The model under review builds one solid part; all positions refer to its coordinate system, in mm. A direction names the side the tool comes from. Give positions to 0.01 mm unless a question says otherwise; leave off trailing zeros. Loops run counter-clockwise (first coordinate to the right, second up) from the corner with the lowest first, then second, coordinate; pieces in that order, holes last. Notation, with made-up numbers: M -8,68 L 18,68 A11 cw 18,77 Z; hole C 82,-16 d4. An arc over 180 degrees is marked long. Write item = value, one per line. Start each with the question number.
1. We need section C-C on x = 0. Give the boundary of the cut face in (y, z), then the cut area to 3 significant figures.
2. Wall thickness on line 1 along X through (y, z) = (5.5, -5); line 2 along Z through (x, y) = (-8.5, 7); line 3 along Z through (x, y) = (3.25, 4): over which ranges is each line inside the solid? List them lowest first. Write a range as from..to.
3. For pin 1 (5 mm diameter, centred on x = -7.5, z = -8.5, fed in from +Y); pin 2 (6 mm diameter, centred on x = 6.5, y = 11, fed in from +Z); pin 3 (3.5 mm diameter, centred on x = -13, z = 16, fed in from +Y); pin 4 (5 mm diameter, centred on y = 22, z = -0.5, fed in from -X), all flat-tipped, find the tip position at first contact; note any pin that passes through.
4. We need section A-A on y = 21. Give the boundary of the cut face in (x, z).
5. For faces 1 (the face through (4.4, 2, 1)), 2 (the face through (-13, 6.8, 15)), 3 (the face through (-11, 13, -5)), list the 3-axis set-ups (+Z, -Z, +X, -X, +Y, -Y) from which the entire face can be reached by the end or side of a thin tool; tool diameter is ignored.
6. We need section D-D on z = -13.5. Give the boundary of the cut face in (x, y), then the cut area to 3 significant figures.
7. Draft analysis for pull direction X (two halves, no side actions). For faces 4 (the face through (6, 17, -17.5)), 5 (the face through (14, 13, -4)), 6 (the face through (-4.4, 2, 1)), 7 (the face through (-14, 13, -4)), state which applies: pulls with the +X half, pulls with the -X half, needs draft (parallel to the pull), parting line crosses it, or undercut.
8. We need section B-B on z = 5. Give the boundary of the cut face in (x, y), then the cut area to 3 significant figures.
Autodesk Inventor part; units mm, degrees
ref_plane "YZ Plane" through (0, 0, 0) normal (1, 0, 0) x (0, 1, 0)
ref_plane "XZ Plane" through (0, 0, 0) normal (0, 1, 0) x (-1, 0, 0)
ref_plane "XY Plane" through (0, 0, 0) normal (0, 0, 1) x (1, 0, 0)
sketch "Sketch1" plane through (0, 0, 0) normal (0, 1, 0) x (-1, 0, 0)
  line L0 (14, 17.5) -> (-14, 17.5)
  line L1 (-14, 17.5) -> (-14, -17.5)
  line L2 (-14, -17.5) -> (14, -17.5)
  line L3 (14, -17.5) -> (14, 17.5)
  point P0 (0, 0)
  dimension "d0" = 35
  dimension "d1" = 28
  dimension "d2" = 14
  dimension "d3" = 17.5
extrude "Extrusion1" add sketch "Sketch1" along normal blind 4.5
sketch "Sketch2" plane through (14, 0, 17.5) normal (1, 0, 0) x (0, 0, -1)
  line L0 (0, 0) -> (35, 0)
  line L1 (35, 0) -> (35, 4.5)
  line L2 (0, 4.5) -> (35, 4.5)
  line L3 (0, 0) -> (0, 4.5)
  line L4 (35, 0) -> (35, 35)
  line L5 (35, 35) -> (28.2, 35)
  line L6 (28.2, 35) -> (28.2, 30)
  line L7 (28.2, 30) -> (5, 6.8)
  line L8 (5, 6.8) -> (0, 6.8)
  line L9 (0, 0) -> (35, 0)
  line L10 (0, 6.8) -> (0, 0)
  point P0 (17.5, 0)
  point P1 (0, 4.5)
  dimension "d6" = 6.8
  dimension "d7" = 5
extrude "Extrusion2" add sketch "Sketch2" against normal blind 3 contours L10 L8 L7 L6 L5 L4 L2
sketch "Sketch3" plane through (-14, 0, -17.5) normal (-1, 0, 0) x (0, 0, 1)
  line L0 (35, 4.5) -> (35, 6.8)
  line L1 (35, 6.8) -> (30, 6.8)
  line L2 (30, 6.8) -> (6.8, 30)
  line L3 (6.8, 30) -> (6.8, 35)
  line L4 (6.8, 35) -> (0, 35)
  line L5 (0, 35) -> (0, 4.5)
  line L6 (35, 4.5) -> (0, 4.5)
  line L7 (0, 0) -> (35, 0)
  line L8 (35, 0) -> (35, 4.5)
  line L9 (0, 4.5) -> (35, 4.5)
  line L10 (0, 0) -> (0, 4.5)
  point P0 (17.5, 0)
  point P1 (0, 4.5)
extrude "Extrusion3" add sketch "Sketch3" against normal blind 3
sketch "Sketch4" plane through (14, 0, -17.5) normal (0, 0, -1) x (-1, 0, 0)
  line L0 (3, 4.5) -> (25, 4.5)
  line L1 (3, 35) -> (3, 4.5)
  line L2 (0, 35) -> (3, 35)
  line L3 (0, 0) -> (0, 35)
  line L4 (0, 0) -> (28, 0)
  line L5 (28, 0) -> (28, 35)
  line L6 (28, 35) -> (25, 35)
  line L7 (25, 4.5) -> (25, 35)
  line L8 (0, 35) -> (3, 35)
  line L9 (28, 30) -> (28, 35)
  line L10 (0, 35) -> (28, 35)
  point P0 (14, 0)
  point P1 (25, 35)
extrude "Extrusion4" add sketch "Sketch4" against normal blind 4.5
sketch "Sketch5" plane through (0, 4.5, 0) normal (0, 1, 0) x (1, 0, 0)
  line L0 (14, -17.5) -> (14, 17.5)
  line L1 (-14, -17.5) -> (14, -17.5)
  line L2 (-14, 17.5) -> (-14, -17.5)
  line L3 (14, 17.5) -> (-14, 17.5)
  line L4 (11, 13) -> (-11, 13)
  line L5 (-11, 13) -> (-11, -17.5)
  line L6 (-11, -17.5) -> (11, -17.5)
  line L7 (11, -17.5) -> (11, 13)
  line L8 (0, 3.5) -> (0, -5.5) construction
  line L9 (-4.4, 3.5) -> (-4.4, -5.5)
  line L10 (4.4, -5.5) -> (4.4, 3.5)
  arc A0 (4.4, 3.5) -> (-4.4, 3.5) centre (0, 3.5) ccw
  arc A1 (-4.4, -5.5) -> (4.4, -5.5) centre (0, -5.5) ccw
  point P0 (0, 0)
  point P1 (0, -1)
  dimension "d14" = 14
  dimension "d15" = 9
  dimension "d16" = 8.8
extrude "Extrusion5" cut sketch "Sketch5" against normal through all contours A0 L10 A1 L9
sketch "Sketch6" plane through (14, 0, -13) normal (0, 0, 1) x (1, 0, 0)
  line L0 (-14, 23) -> (-14, 14) construction
  line L1 (-18.4, 23) -> (-18.4, 14)
  line L2 (-9.6, 14) -> (-9.6, 23)
  arc A0 (-9.6, 23) -> (-18.4, 23) centre (-14, 23) ccw
  arc A1 (-18.4, 14) -> (-9.6, 14) centre (-14, 14) ccw
  line L3 (-28, 0) -> (0, 0)
  line L4 (-14, 7.4113) -> (0, 7.4113) construction
  line L5 (0, 30) -> (0, 6.8)
  point P0 (-14, 0)
  point P1 (-14, 18.5)
  dimension "d19" = 9
  dimension "d20" = 8.8
  dimension "d21" = 14
  dimension "d22" = 14
extrude "Extrusion6" cut sketch "Sketch6" against normal blind 10
properties part number "3030_angle"
Final values:
q1.outline = M 0,-17.5 L 9.6,-17.5 L 9.6,-13 L 4.5,-13 L 4.5,-7.9 L 0,-7.9 Z; M 0,9.9 L 4.5,9.9 L 4.5,17.5 L 0,17.5 Z; M 27.4,-17.5 L 35,-17.5 L 35,-13 L 27.4,-13 Z
q1.area = 135 mm²
q2.line_1 = -14..-11, 11..14
q2.line_2 = -17.5..-13
q2.line_3 = -17.5..-6.47, 8.47..17.5
q3.pin_1 = 4.5
q3.pin_2 = -13
q3.pin_3 = 6.8
q3.pin_4 = -14
q4.outline = M -14,-17.5 L -4.4,-17.5 L -4.4,-13 L -11,-13 L -11,-1.7 L -14,-1.7 Z; M 4.4,-17.5 L 14,-17.5 L 14,-1.7 L 11,-1.7 L 11,-13 L 4.4,-13 Z
q5.face_1 = +Y, -Y
q5.face_2 = +Z, +X, -X, +Y
q5.face_3 = +Z, +Y
q6.outline = M -14,0 L 14,0 L 14,35 L -14,35 Z; hole M -4.4,14 A4.4 ccw 4.4,14 L 4.4,23 A4.4 ccw -4.4,23 Z
q6.area = 840 mm²
q7.face_4 = needs draft
q7.face_5 = pulls with the +X half
q7.face_6 = undercut
q7.face_7 = pulls with the -X half
q8.outline = M -14,0 L -4.4,0 L -4.4,4.5 L -11,4.5 L -11,14.3 L -14,14.3 Z; M 4.4,0 L 14,0 L 14,14.3 L 11,14.3 L 11,4.5 L 4.4,4.5 Z
q8.area = 145 mm²
